The model under review builds one solid part; all positions refer to its coordinate system, in mm. A direction names the side the tool comes from. Give positions to 0.01 mm unless a question says otherwise; leave off trailing zeros. Write each loop counter-clockwise with the first axis right and the second up, starting at its lowest first coordinate (ties: lowest second). Pieces come first, ordered by that corner, then holes. Notation, with made-up numbers: (81.5, 20) -> (95.5, 20) arc R30 ccw to (95.5, 55) -> close; hole circle Ø7 at (68.5, 8). An arc over 180 degrees is marked (long way). Use CSV: the item, a comma, the result in double quotes.
```python
from build123d import *

# Parameters (mm, degrees)
PAD003_DEPTH    = 7.5
SKETCH005_R     = 1
POCKET001_DEPTH = 7.001
CHAMFER003_SIZE = 1
CHAMFER007_SIZE = 1


with BuildPart() as part:
    # Sketch004 → Pad003 (new body, symmetric)
    with BuildSketch(Plane.XY):
        Polygon((0, 0), (0, -8), (3.25, -8), (3.25, -23.5), (0, -23.5), (0, -31.5), (7, -31.5), (7, 7), align=None)
    extrude(amount=PAD003_DEPTH, both=True)

    # Sketch005 (on Face7 of Pad003) → Pocket001 (cut, through all)
    with BuildSketch(Plane.YZ.offset(7)):
        with Locations((-26.5, 0)):
            Circle(SKETCH005_R)
        with Locations((-5, 0)):
            Circle(SKETCH005_R)
    extrude(amount=-POCKET001_DEPTH, mode=Mode.SUBTRACT)

    # Chamfer003
    chamfer003_edges = [part.edges().sort_by_distance(p)[0] for p in [
        (7, -27.5, 0),
        (7, -6, 0),
    ]]
    chamfer(chamfer003_edges, length=CHAMFER003_SIZE)

    # Chamfer007
    chamfer007_edges = [part.edges().sort_by_distance(p)[0] for p in [
        (7, -12.25, -7.5),
        (7, -31.5, 0),
        (7, -12.25, 7.5),
    ]]
    chamfer(chamfer007_edges, length=CHAMFER007_SIZE)


solid = part.part
```
Q1. Insertion check: pin 1 (3.5 mm diameter, centred on x = 1, z = -3.5, fed in from +Y); pin 2 (1 mm diameter, centred on x = 4, z = -6, fed in from +Y); pin 3 (1 mm diameter, centred on x = 5.5, z = 2.5, fed in from +Y); pin 4 (1.8 mm diameter, centred on y = -5, z = 0, fed in from +X). Each pin has a flat end and moves straight along its axis. Give the tip position at first contact, or say it passes through.
Derived:
pin 1,"stops at y = 2.75"
pin 2,"stops at y = 4.5"
pin 3,"stops at y = 6"
pin 4,"passes through"
Q2. Machinability: for faces 4 (the flat face through (4, -12, 7.5)), 5 (the flat face through (2, -8, 0)), which of the approach directions +Z, -Z, +X, -X, +Y, -Y give a long, thin tool a straight path to every point of the face, cutting with its end or side? Answer none if there is none.
Derived:
face 4,"+Z, +X, -X, +Y, -Y"
face 5,"+Z, -Z, -X"
Q3. Consider section A-A (x = 2.5). Write out the cut boundary in (y, z), then the cut area to 3 significant figures.
Derived:
outline,"(-31.5, -7.5) -> (-23.5, -7.5) -> (-23.5, 7.5) -> (-31.5, 7.5) -> close; (-8, -7.5) -> (2.5, -7.5) -> (2.5, 7.5) -> (-8, 7.5) -> close; hole circle Ø2 at (-26.5, 0); hole circle Ø2 at (-5, 0)"
area,"271 mm2"
Q4. Consider section B-B (y = -5). Write out the cut boundary in (x, z).
Derived:
outline,"(0, -7.5) -> (6, -7.5) -> (7, -6.5) -> (7, -2) -> (6, -1) -> (0, -1) -> close; (0, 1) -> (6, 1) -> (7, 2) -> (7, 6.5) -> (6, 7.5) -> (0, 7.5) -> close"
Q5. Consider section D-D (x = 4). Write out the cut boundary in (y, z).
Derived:
outline,"(-31.5, -7.5) -> (4, -7.5) -> (4, 7.5) -> (-31.5, 7.5) -> close; hole circle Ø2 at (-26.5, 0); hole circle Ø2 at (-5, 0)"
Q6. Consider section C-C (z = 0). Write out the cut boundary in (x, y).
Derived:
outline,"(0, -31.5) -> (6, -31.5) -> (7, -30.5) -> (7, -28.5) -> (6, -27.5) -> (0, -27.5) -> close; (0, -25.5) -> (6, -25.5) -> (7, -24.5) -> (7, -7) -> (6, -6) -> (0, -6) -> (0, -8) -> (3.25, -8) -> (3.25, -23.5) -> (0, -23.5) -> close; (0, -4) -> (6, -4) -> (7, -3) -> (7, 7) -> (0, 0) -> close"
Q7. The part is to be moulded in two halves that separate along Y. For faces 1 (the flat face through (3, -31.5, 0)), 2 (the cylindrical face through (3, -27.5, 0)), 3 (the flat face through (0, -28, 0)), say which applies: pulls with the +Y half, pulls with the -Y half, needs draft (parallel to the pull), parting line crosses it, or undercut.
Derived:
face 1,"pulls with the -Y half"
face 2,"undercut"
face 3,"needs draft"
Q8. To check wall thickness, follow probe 1 along Y at (x, z) = (2, -3.25); probe 2 along Z at (x, y) = (2.8, -26.5); probe 3 along X at (y, z) = (-16, -5.25). State the ranges of each line that lie inside material, in increasing order.
Derived:
probe 1,"y = -31.5 to -23.5, -8 to 2"
probe 2,"z = -7.5 to -1, 1 to 7.5"
probe 3,"x = 3.25 to 7"
